Part model, mm, in its own coordinate system. A direction names the side the tool comes from. Round coordinates to 2 decimals unless told otherwise and drop trailing zeros. Write each loop counter-clockwise with the first axis right and the second up, starting at its lowest first coordinate (ties: lowest second). Pieces come first, ordered by that corner, then holes. Notation, with made-up numbers: (-39, -11) -> (1, -11) arc R23 cw to (1, 28) -> close; hole circle Ø3 at (-26.75, 7.25). An arc over 180 degrees is marked (long way). Use CSV: the item, a comma, the result in double quotes. Start each with the question number.
(1) Drop flat-ended pins along their axis: pin 1 (2 mm diameter, centred on x = 0, z = 0, fed in from -Y); pin 2 (2 mm diameter, centred on y = -3, z = 2.5, fed in from -X); pin 3 (4 mm diameter, centred on y = -12, z = -3, fed in from -X). Give the stop position or say it passes through.
(2) Saw through at C-C (z = -1.75). Give the cut face in (x, y).
(3) Saw through at A-A (x = 0). Give the cut face in (y, z) (3 decimals), plus the area to 3 significant figures.
(4) Saw through at D-D (x = 1.5). Give the cut face in (y, z).
(5) Saw through at B-B (z = 0). Give the cut face in (x, y) (3 decimals), plus the area to 3 significant figures.
(6) Probe line 1 (Z direction, x = 0, y = -8.5); line 2 (Z direction, x = 0, y = -3.5) (3 decimals); line 3 (Y direction, x = 1.25, z = -2). List the from-to ranges inside material, lowest first. Write a range as [from, to].
(7) Two-plate mould, pull along X, no slides. Class faces 4 (the flat face through (2.4, -19.7, -2.4)), 5 (the flat face through (-1, -6, -1)), 6 (the cylindrical face through (-1.19, -9.71, -5.37)): released by +X, released by -X, zero draft, split by the parting line, or undercut.
(8) Which spindle directions (+Z, -Z, +X, -X, +Y, -Y) get a long thin tool onto all of the face, cutting with end or side? Do faces 1 (the cylindrical face through (0.69, -2.96, -3.1)), 2 (the cylindrical face through (-0.69, -16.1, -3.1)), 3 (the cylindrical face through (-0.63, -9.24, -0.49)). Say none if no direction does.
```python
from build123d import *

# Parameters (mm, degrees)
F0_R     = 5.5
F1_DEPTH = 19.7
F2_R     = 3.175
F3_DEPTH = 7.3
F5_R     = 3.175
F6_DEPTH = 6
F4_R     = 0.8
F7_DEPTH = 12.401


with BuildPart() as f1:
    # F0 (on Front) → F1 (new body)
    with BuildSketch(Plane.XZ):
        Circle(F0_R)
    extrude(amount=F1_DEPTH)

    # F2 (on face) → F3 (cut)
    with BuildSketch(Plane.XZ.offset(19.7)):
        Circle(F2_R)
    extrude(amount=-F3_DEPTH, mode=Mode.SUBTRACT)

    # F5 (on face) → F6 (cut)
    with BuildSketch(Plane(origin=(0, 0, 0), x_dir=(-1, 0, 0), z_dir=(0, 1, 0))):
        Circle(F5_R)
    extrude(amount=-F6_DEPTH, mode=Mode.SUBTRACT)

    # F4 (on face) → F7 (cut, through all)
    with BuildSketch(Plane.XZ.offset(12.4)):
        Circle(F4_R)
    extrude(amount=-F7_DEPTH, mode=Mode.SUBTRACT)


solid = f1.part
```
Answers:
1,pin 1,"stops at y = -12.4"
1,pin 2,"stops at x = -5.29"
1,pin 3,"stops at x = -5.41"
2,outline,"(-5.21, -19.7) -> (-2.65, -19.7) -> (-2.65, -12.4) -> (2.65, -12.4) -> (2.65, -19.7) -> (5.21, -19.7) -> (5.21, 0) -> (2.65, 0) -> (2.65, -6) -> (-2.65, -6) -> (-2.65, 0) -> (-5.21, 0) -> close"
3,outline,"(-19.7, -5.5) -> (0, -5.5) -> (0, -3.175) -> (-6, -3.175) -> (-6, -0.8) -> (-12.4, -0.8) -> (-12.4, -3.175) -> (-19.7, -3.175) -> close; (-19.7, 3.175) -> (-12.4, 3.175) -> (-12.4, 0.8) -> (-6, 0.8) -> (-6, 3.175) -> (0, 3.175) -> (0, 5.5) -> (-19.7, 5.5) -> close"
3,area,"122 mm²"
4,outline,"(-19.7, -5.29) -> (0, -5.29) -> (0, -2.8) -> (-6, -2.8) -> (-6, 2.8) -> (0, 2.8) -> (0, 5.29) -> (-19.7, 5.29) -> (-19.7, 2.8) -> (-12.4, 2.8) -> (-12.4, -2.8) -> (-19.7, -2.8) -> close"
5,outline,"(-5.5, -19.7) -> (-3.175, -19.7) -> (-3.175, -12.4) -> (-0.8, -12.4) -> (-0.8, -6) -> (-3.175, -6) -> (-3.175, 0) -> (-5.5, 0) -> close; (0.8, -12.4) -> (3.175, -12.4) -> (3.175, -19.7) -> (5.5, -19.7) -> (5.5, 0) -> (3.175, 0) -> (3.175, -6) -> (0.8, -6) -> close"
5,area,"122 mm²"
6,line 1,"z = [-5.5, -0.8], [0.8, 5.5]"
6,line 2,"z = [-5.5, -3.175], [3.175, 5.5]"
6,line 3,"y = [-12.4, -6]"
7,face 4,"zero draft"
7,face 5,"undercut"
7,face 6,"split by the parting line"
8,face 1,"+Y"
8,face 2,"-Y"
8,face 3,"+Y, -Y"
